Here's how the part is built. I have some questions about the finished solid (model axes, mm). Face numbers are marked on the shaded views. Round coordinates to 2 decimals unless told otherwise and drop trailing zeros. Write each loop counter-clockwise with the first axis right and the second up, starting at its lowest first coordinate (ties: lowest second). Pieces come first, ordered by that corner, then holes. Notation, with made-up numbers: (75, -10.5) -> (108, -10.5) arc R20 cw to (108, 11.5) -> close; hole circle Ø10 at (81.5, -3). An arc over 180 degrees is marked (long way). Put each result on its own line as item: value. Start each with the question number.
1. I need wall thicknesses on probe 1 along Z at (x, y) = (0, -3.25); probe 2 along Z at (x, y) = (0, -10); probe 3 along X at (y, z) = (25.5, -1.75). Which ranges of each line are inside material? Lowest first, please. Write a range as from..to.
2. Suppose I cut it at C-C (z = 0). Please give me the cut outline in (x, y).
3. Suppose I cut it at A-A (x = 0). Please give me the cut outline in (y, z).
4. Suppose I cut it at B-B (y = 22). Please give me the cut outline in (x, z).
5. Suppose I cut it at D-D (y = -8.5). Please give me the cut outline in (x, z), then the cut area to 3 significant figures.
6. For pin 1 (5 mm diameter, centred on x = 32, y = 26.5, fed in from +Z); pin 2 (4 mm diameter, centred on x = -21.5, z = -0.5, fed in from -Y); pin 3 (4.5 mm diameter, centred on x = -1, z = -0.5, fed in from -Y); pin 4 (3 mm diameter, centred on y = 24, z = 1, fed in from -X), each with a flat end and sliding along its axis, tell me the tip position at first contact or that it passes through.
7. We'd pull the mould along Y, two halves only. Please class the marked faces 1, 2 and 3: +Y half, -Y half, draft (parallel to the pull), parting line (faces both ways), or undercut.
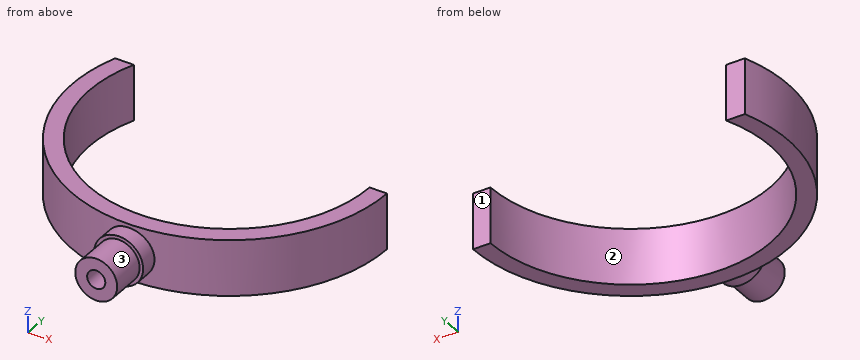
```python
from build123d import *

# Parameters (mm, degrees)
PAD_DEPTH     = 8
SKETCH002_R   = 7
PAD001_DEPTH  = 4.5
POCKET_DEPTH  = 5
SKETCH005_R   = 6
SKETCH005_R_2 = 2.6
PAD002_DEPTH  = 10


with BuildPart() as part:
    # Sketch001 → Pad (new body, symmetric)
    with BuildSketch(Plane.XY):
        with BuildLine():
            ThreePointArc((-37.080992, 60), (-7.64069, 5.736533), (40, 45))
            Line((40, 45), (45, 45))
            ThreePointArc((-42.426407, 60), (-7.609589, 0.648065), (45, 45))
            Line((-42.426407, 60), (-37.080992, 60))
        make_face()
    extrude(amount=PAD_DEPTH, both=True)

    # Sketch002 → Pad001 (join, symmetric)
    with BuildSketch(Plane.XZ):
        Circle(SKETCH002_R)
    extrude(amount=PAD001_DEPTH, both=True)

    # Sketch004 (on Face8 of Pad001) → Pocket (cut)
    with BuildSketch(Plane.XZ.offset(4.5)):
        with BuildLine():
            Line((-1.532971, 2.1), (1.532971, 2.1))
            ThreePointArc((1.532971, -2.1), (2.6, 0), (1.532971, 2.1))
            Line((-1.532971, -2.1), (1.532971, -2.1))
            ThreePointArc((-1.532971, 2.1), (-2.6, 0), (-1.532971, -2.1))
        make_face()
    extrude(amount=-POCKET_DEPTH, mode=Mode.SUBTRACT)

    # Sketch005 (on Face8 of Pocket) → Pad002 (join)
    with BuildSketch(Plane.XZ.offset(4.5)):
        Circle(SKETCH005_R)
        Circle(SKETCH005_R_2, mode=Mode.SUBTRACT)
    extrude(amount=PAD002_DEPTH)


solid = part.part
```
Verdict:
1. probe 1: z = -7..-2.1, 2.1..7
1. probe 2: z = -6..-2.6, 2.6..6
1. probe 3: x = -40.56..-34.92, 34.92..40.56
2. outline: (-42.43, 60) arc R45 ccw to (-7, 0.55) -> (-7, -4.5) -> (-6, -4.5) -> (-6, -14.5) -> (-2.6, -14.5) -> (-2.6, 0.5) -> (2.6, 0.5) -> (2.6, -14.5) -> (6, -14.5) -> (6, -4.5) -> (7, -4.5) -> (7, 0.55) arc R45 ccw to (45, 45) -> (40, 45) arc R40 cw (long way) to (-37.08, 60) -> close
3. outline: (-14.5, -6) -> (-4.5, -6) -> (-4.5, -7) -> (0, -7) -> (0, -8) -> (5, -8) -> (5, 8) -> (0, 8) -> (0, 7) -> (-4.5, 7) -> (-4.5, 6) -> (-14.5, 6) -> (-14.5, 2.6) -> (-4.5, 2.6) -> (-4.5, 2.1) -> (0.5, 2.1) -> (0.5, -2.1) -> (-4.5, -2.1) -> (-4.5, -2.6) -> (-14.5, -2.6) -> close
4. outline: (-38.68, -8) -> (-32.73, -8) -> (-32.73, 8) -> (-38.68, 8) -> close; (32.73, -8) -> (38.68, -8) -> (38.68, 8) -> (32.73, 8) -> close
5. outline: circle Ø12 at (0, 0); hole circle Ø5.2 at (0, 0)
5. area: 91.9 mm^2
6. pin 1: passes through
6. pin 2: stops at y = 4.44
6. pin 3: stops at y = -14.5
6. pin 4: stops at x = -40.56
7. face 1: +Y half
7. face 2: undercut
7. face 3: draft
